Drawing for the job (mm, zero at the part's lowest x, y, z). Coordinates: 2 decimals unless noted, no trailing zeros. Order: outer loops, then holes, each group sorted by start corner. A loop starts at its lowest first (then second) coordinate and runs counter-clockwise, first axis right, second up. Notation, with made-up numbers: (-6.75, -13.5) - (39.25, -13.5) arc R24 cw to (39.25, 1.5) - close; hole circle Ø9 at (86.5, 36). An arc over 180 degrees is marked (long way). Answer as CSV lines item,"result". Start each with the question number.
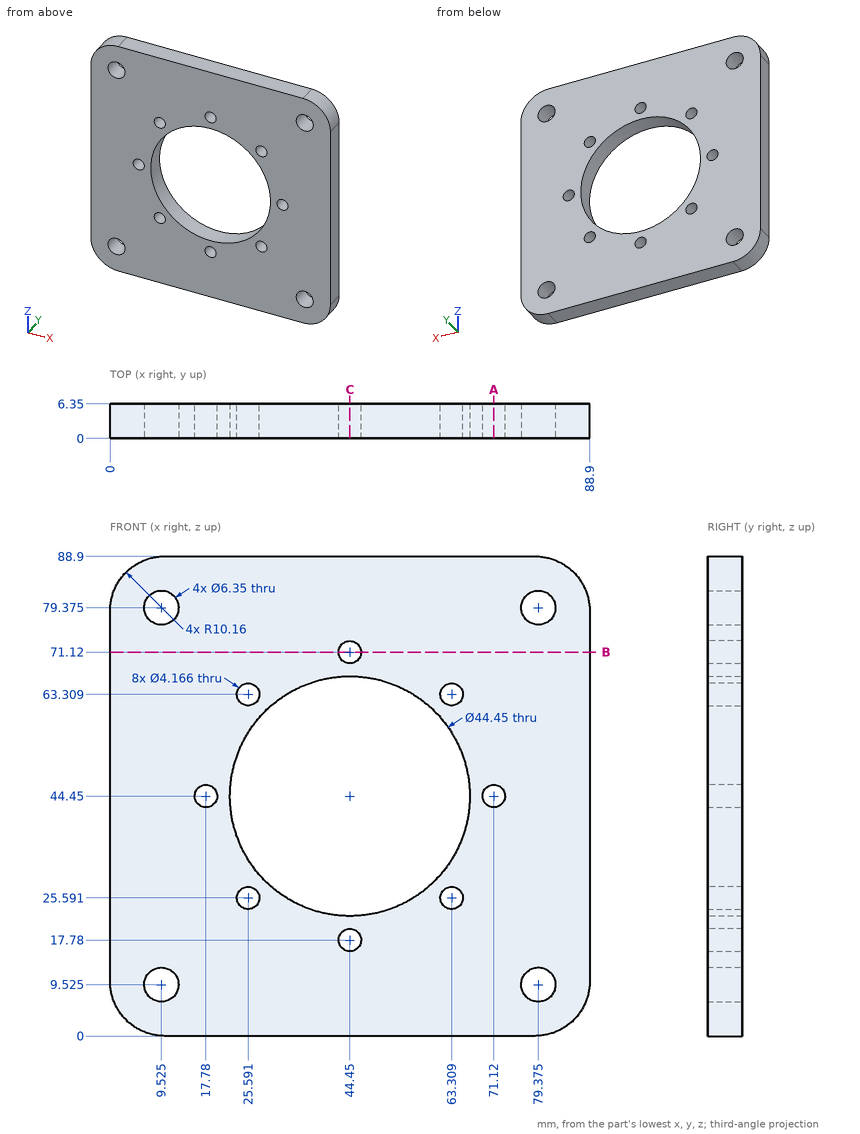
(1) Probe L1, parallel to Z at x = 59, y = 3.5; L2, parallel to X at y = 2.25, z = 44.45 (1 decimal); L3, parallel to X at y = 1.5, z = 17.78. List the from-to ranges inside material, lowest first. Write a range as [from, to].
(2) Band-saw the part on B-B on z = 71.12. List the corners of the cut face in (x, y).
(3) Band-saw the part on A-A on x = 71.12. List the corners of the cut face in (y, z).
(4) Band-saw the part on C-C on x = 44.45. State how many separate pieces and enclosed holes the cut face has, plus the area to 3 significant figures.
Filled in:
1,L1,"z = [0, 27.65], [61.25, 88.9]"
1,L2,"x = [0, 15.7], [19.9, 22.2], [66.7, 69], [73.2, 88.9]"
1,L3,"x = [0, 42.37], [46.53, 88.9]"
2,outline,"(0, 0) - (42.37, 0) - (42.37, 6.35) - (0, 6.35) - close; (46.53, 0) - (88.9, 0) - (88.9, 6.35) - (46.53, 6.35) - close"
3,outline,"(0, 0) - (6.35, 0) - (6.35, 42.37) - (0, 42.37) - close; (0, 46.53) - (6.35, 46.53) - (6.35, 88.9) - (0, 88.9) - close"
4,separate pieces,"4"
4,enclosed holes,"0"
4,area,"229 mm^2"
